from build123d import *

# Parameters (mm, degrees)
SALIENTE_EXTRUIR1_DEPTH      = 10
SALIENTE_EXTRUIR1_DEPTH_BACK = 10
CROQUIS1_R                   = 10.25
CROQUIS1_R_2                 = 6.25
CROQUIS2_R                   = 1.55
CORTAR_EXTRUIR1_DEPTH        = 8.5
CROQUIS3_R                   = 1.55
CORTAR_EXTRUIR2_DEPTH        = 28.5


with BuildPart() as part:
    # Croquis1 → Saliente-Extruir1 (new, two sides: drawn at the far end of the back side and taken through both)
    with BuildSketch(Plane.XY.offset(-SALIENTE_EXTRUIR1_DEPTH_BACK)):
        Circle(CROQUIS1_R)
        Circle(CROQUIS1_R_2, mode=Mode.SUBTRACT)
    extrude(amount=SALIENTE_EXTRUIR1_DEPTH + SALIENTE_EXTRUIR1_DEPTH_BACK)

    # Croquis2 → Cortar-Extruir1 (cut)
    # profile 1 of 2: a face of its own
    with BuildSketch(Plane(origin=(0, 0, 0), x_dir=(1, 0, 0), z_dir=(0, 1, 0))):
        Polygon((1.529978213, -2.35), (-1.529978213, -2.35), (-3.059956427, -5), (-1.529978213, -7.65), (1.529978213, -7.65), (3.059956427, -5), align=None)
        with Locations(Location((0, -5, 0), (0, 0, 270))):
            Circle(CROQUIS2_R, mode=Mode.SUBTRACT)
    # profile 2 of 2: a face of its own
    with BuildSketch(Plane(origin=(0, 0, 0), x_dir=(1, 0, 0), z_dir=(0, 1, 0))):
        Polygon((3.059956427, 5), (1.529978213, 2.35), (-1.529978213, 2.35), (-3.059956427, 5), (-1.529978213, 7.65), (1.529978213, 7.65), align=None)
        with Locations(Location((0, 5, 0), (0, 0, 270))):
            Circle(CROQUIS2_R, mode=Mode.SUBTRACT)
    extrude(amount=-CORTAR_EXTRUIR1_DEPTH, mode=Mode.SUBTRACT)

    # Croquis3 → Cortar-Extruir2 (cut)
    with BuildSketch(Plane(origin=(0, 0, 0), x_dir=(1, 0, 0), z_dir=(0, 1, 0))):
        with Locations(Location((0, 5, 0), (0, 0, 270))):
            Circle(CROQUIS3_R)
        with Locations(Location((0, -5, 0), (0, 0, 270))):
            Circle(CROQUIS3_R)
    extrude(amount=-CORTAR_EXTRUIR2_DEPTH, mode=Mode.SUBTRACT)


solid = part.part
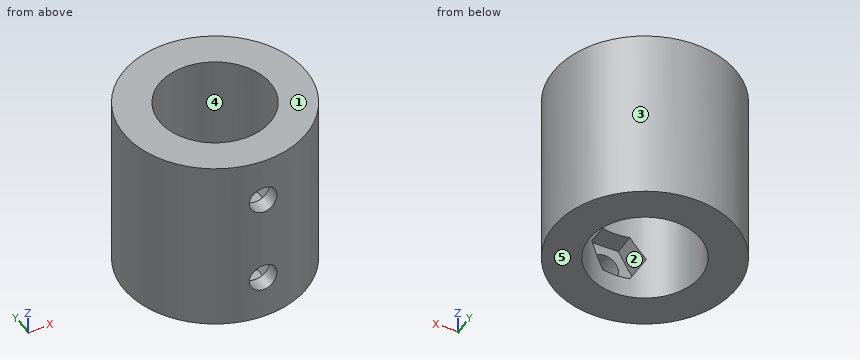
Geometry check sheet. Reference: the model listing, model coordinates, mm. Face numbers are marked on the shaded views. A direction names the side the tool comes from. Give positions to 0.01 mm unless a question says otherwise; leave off trailing zeros. Loops run counter-clockwise (first coordinate to the right, second up) from the corner with the lowest first, then second, coordinate; pieces in that order, holes last. Notation, with made-up numbers: (-29, 28) -> (2, 28) arc R10 ccw to (2, 44) -> close; hole circle Ø2 at (38, 58). An arc over 180 degrees is marked (long way). Answer in a Markdown table with one row per item. Add a question column.
1) Set-up check for the marked faces 1 and 2: record each of +Z, -Z, +X, -X, +Y, -Y from which the full face is reachable in a straight line by a thin tool's end or side.
2) Draft check along X on the marked faces 3, 4 and 5. Enter one of: pulls with the +X half, pulls with the -X half, needs draft (parallel to the pull), parting line crosses it, or undercut.
3) Material ranges on probe 1 along Z at (x, y) = (0, -9.4); probe 2 along X at (y, z) = (-5, -1.5); probe 3 along Y at (x, z) = (3.25, -2.5), recorded low to high. Write a range as from..to.
4) Cross-section at B-B on y = 0. Record the boundary of the cut face in (x, z), and give its area (3 significant figures).
5) Cross-section at A-A on x = 0. Record the boundary of the cut face in (y, z), and give its area (3 significant figures).
6) Cross-section at C-C on z = 0.5. Record the boundary of the cut face in (x, y).
7) Gauge pin test, flat ends, axial feed: P1, Ø1.5, axis at x = -7, z = 2.5, coming from the +Y side; P2, Ø2, axis at y = 4.5, z = -2, coming from the +X side; P3, Ø1, axis at x = -4, z = -1, coming from the +Y side. Record the tip position at first contact, or that the pin passes through.
8) Cross-section at D-D on x = -5. Record the boundary of the cut face in (y, z).
Outcome:
| question | item | result |
|---|---|---|
| 1 | face 1 | +Z, +X, -X, +Y, -Y |
| 1 | face 2 | none |
| 2 | face 3 | parting line crosses it |
| 2 | face 4 | undercut |
| 2 | face 5 | needs draft |
| 3 | probe 1 | z = -10..-6.55, -3.45..3.45, 6.55..10 |
| 3 | probe 2 | x = -8.95..-3.75, 3.75..8.95 |
| 3 | probe 3 | y = -9.72..-5.34, 5.34..9.72 |
| 4 | outline | (-10.25, -10) -> (-6.25, -10) -> (-6.25, 10) -> (-10.25, 10) -> close; (6.25, -10) -> (10.25, -10) -> (10.25, 10) -> (6.25, 10) -> close |
| 4 | area | 160 mm^2 |
| 5 | outline | (-10.25, -10) -> (-6.25, -10) -> (-6.25, -7.65) -> (-8.5, -7.65) -> (-8.5, -6.55) -> (-10.25, -6.55) -> close; (-10.25, -3.45) -> (-8.5, -3.45) -> (-8.5, -2.35) -> (-6.25, -2.35) -> (-6.25, 2.35) -> (-8.5, 2.35) -> (-8.5, 3.45) -> (-10.25, 3.45) -> close; (-10.25, 6.55) -> (-8.5, 6.55) -> (-8.5, 7.65) -> (-6.25, 7.65) -> (-6.25, 10) -> (-10.25, 10) -> close; (6.25, -10) -> (10.25, -10) -> (10.25, 10) -> (6.25, 10) -> close |
| 5 | area | 125 mm^2 |
| 6 | outline | circle Ø20.5 at (0, 0); hole circle Ø12.5 at (0, 0) |
| 7 | P1 | stops at y = 8.12 |
| 7 | P2 | stops at x = 9.63 |
| 7 | P3 | stops at y = 9.63 |
| 8 | outline | (-8.95, -10) -> (-3.75, -10) -> (-3.75, 10) -> (-8.95, 10) -> close; (3.75, -10) -> (8.95, -10) -> (8.95, 10) -> (3.75, 10) -> close |
